```python
from build123d import *

# Parameters (mm, degrees)
SKETCH1_W                      = 101.6
SKETCH1_H                      = 42.727601577
BOSS_EXTRUDE2_DEPTH            = 6
M3_CLEARANCE_HOLE1_D           = 3.4
M3_CLEARANCE_HOLE1_CSINK_D     = 3.45
M3_CLEARANCE_HOLE1_CSINK_ANGLE = 90
CUT_EXTRUDE1_DEPTH             = 77.129253004
CUT_EXTRUDE2_DEPTH             = 77.129253004


with BuildPart() as part:
    # Sketch1 → Boss-Extrude2 (new body)
    with BuildSketch(Plane(origin=(0, 0, 0), x_dir=(1, 0, 0), z_dir=(0, 1, 0))):
        with Locations((-9.585511853, -24.606332138)):
            Rectangle(SKETCH1_W, SKETCH1_H)
    extrude(amount=BOSS_EXTRUDE2_DEPTH)

    # Sketch5 → CBORE for M3 Hex Socket Head Cap Screw1 (revolve, cut)
    with BuildSketch(Plane(origin=(-50.044280369, 6, 13.782297963), x_dir=(0, 0, 1), z_dir=(1, 0, 0))):
        Polygon((0, 0), (0, 6), (1.6, 6), (1.6, 3.4), (3.25, 3.4), (3.25, 0.025), (3.275, 0), align=None)
    revolve(axis=Axis((-50.044280369, 12.35, 13.782297963), (0, -1, 0)), mode=Mode.SUBTRACT)

    # Sketch8 → CBORE for M3 Hex Socket Head Cap Screw2 (revolve, cut)
    with BuildSketch(Plane(origin=(-49.834104948, 6, 28.914928265), x_dir=(0, 0, 1), z_dir=(1, 0, 0))):
        Polygon((0, 0), (0, 6), (1.7, 6), (1.7, 3.4), (3.25, 3.4), (3.25, 0.025), (3.275, 0), align=None)
    revolve(axis=Axis((-49.834104948, 12.35, 28.914928265), (0, -1, 0)), mode=Mode.SUBTRACT)

    # M3 Clearance Hole1 (through all)
    with Locations(Plane(origin=(0, 6, 0), x_dir=(1, 0, 0), z_dir=(0, 1, 0))):
        with Locations((-34.176036094, -13.467034832)):
            CounterSinkHole(M3_CLEARANCE_HOLE1_D / 2, M3_CLEARANCE_HOLE1_CSINK_D / 2, counter_sink_angle=M3_CLEARANCE_HOLE1_CSINK_ANGLE)

    # Sketch17 → Cut-Extrude1 (cut, through all)
    with BuildSketch(Plane(origin=(0, 6, 0), x_dir=(1, 0, 0), z_dir=(0, 1, 0))):
        Polygon((-22.828510557, -13.43914031), (-21.847349351, -14.573742746), (-20.374174215, -14.291333434), (-19.882160285, -12.874321687), (-20.863321491, -11.739719251), (-22.336496627, -12.022128562), align=None)
    extrude(amount=-CUT_EXTRUDE1_DEPTH, mode=Mode.SUBTRACT)

    # Sketch18 → Cut-Extrude2 (cut, through all)
    with BuildSketch(Plane(origin=(0, 6, 0), x_dir=(1, 0, 0), z_dir=(0, 1, 0))):
        Polygon((-6.426767494, -13.535213432), (-5.799321109, -12.573792338), (-6.035476891, -11.45029337), (-6.996897984, -10.822846985), (-8.120396952, -11.059002767), (-8.747843337, -12.02042386), (-8.511687556, -13.143922829), (-7.550266462, -13.771369213), align=None)
        Polygon((8.704589907, -13.535213432), (8.955713542, -12.642823133), (8.634342974, -11.773257447), (7.863230836, -11.258660909), (6.936915756, -11.295591908), (6.209218611, -11.869944056), (5.958094976, -12.762334355), (6.279465545, -13.631900041), (7.050577683, -14.146496579), (7.976892762, -14.10956558), align=None)
        Polygon((22.401860914, -13.771369213), (22.795252298, -13.101944907), (22.801227077, -12.32551076), (22.418184314, -11.650111674), (21.748760007, -11.25672029), (20.97232586, -11.250745511), (20.296926775, -11.633788275), (19.903535391, -12.303212581), (19.897560612, -13.079646728), (20.280603376, -13.755045814), (20.950027682, -14.148437198), (21.726461829, -14.154411977), align=None)
        Polygon((34.168977745, -13.977066564), (34.643623673, -13.507650611), (34.867592928, -12.878780301), (34.796525653, -12.215011111), (34.444497593, -11.647810671), (33.881232222, -11.289519984), (33.218291156, -11.211102914), (32.586978002, -11.428090924), (32.112332074, -11.897506877), (31.888362819, -12.526377187), (31.959430094, -13.190146377), (32.311458154, -13.757346817), (32.874723525, -14.115637504), (33.537664591, -14.194054574), align=None)
    extrude(amount=-CUT_EXTRUDE2_DEPTH, mode=Mode.SUBTRACT)


solid = part.part
```
Source: CAD feature listing. Evaluate the final solid. Frame: model axes, mm. A direction names the side the tool comes from. Give positions to 0.01 mm unless a question says otherwise; leave off trailing zeros. Put each result on its own line as item: value. Start each with the question number.
1) Material intervals for probe 1 along X at (y, z) = (4, 30.5); probe 2 along X at (y, z) = (5.25, 30), sorted ascending.
2) Reachability of faces 1 (the face through (-10, 0, 24)), 2 (the face through (-48, 2.6, 28)) from +Z, -Z, +X, -X, +Y, -Y: full face, straight path, thin tool, end or side. Return the list, or none.
3) Cut plane A-A (y = 3.5). State how many separate pieces and enclosed holes the cut face has, then the cut area to 3 significant figures.
4) Contact query for flat-ended pins moving along their axis: P1, Ø2.5, axis at x = -50.04, z = 13.78, coming from the +Y side; P2, Ø4.5, axis at x = -49.83, z = 28.91, coming from the +Y side. Output: stop coordinate, or through.
5) Draft query along X for faces 3 (the face through (-60.386, 3, 25)), 4 (the face through (-10, 6, 24)), 5 (the face through (-46.66, 4.31, 28.21)). Return one class per face: released by +X, released by -X, zero draft, split by the parting line, or undercut.
Results are:
1. probe 1: x = -60.39 to -52.67, -47 to 41.21
1. probe 2: x = -60.39 to -52.9, -46.77 to 41.21
2. face 1: +Z, -Z, +X, -X, -Y
2. face 2: +Y
3. separate pieces: 1
3. enclosed holes: 8
3. area: 4,230 mm2
4. P1: passes through
4. P2: stops at y = 2.6
5. face 3: released by -X
5. face 4: zero draft
5. face 5: undercut
